Design review of the part built by this model. Coordinates are the model's own, in mm. A direction names the side the tool comes from. Round coordinates to 2 decimals unless told otherwise and drop trailing zeros. Write each loop counter-clockwise with the first axis right and the second up, starting at its lowest first coordinate (ties: lowest second). Pieces come first, ordered by that corner, then holes. Notation, with made-up numbers: M 46,33 L 101,33 A21 ccw 101,51 Z; hole C 78,4 d1. An arc over 180 degrees is marked long. One line per question, with ' | ' between items. Start each with the question number.
Item 1: Add section A-A, the plane y = 0. State the section outline as (x, z) points.
Item 2: For L1, parallel to Y at x = 0, z = 108.65; L2, parallel to Y at x = 0, z = 50; L3, parallel to Y at x = 0, z = 1.35, list the stretches that pass through material, from the lowest coordinate up.
Item 3: Insertion check: pin 1 Ø3 at (x, z) = (11, 83) entering from +Y; pin 2 Ø10 at (x, z) = (8.5, 54) entering from -Y; pin 3 Ø1 at (y, z) = (6.5, 40.5) entering from +X. Each pin has a flat end and moves straight along its axis. Give the tip position at first contact, or say it passes through.
Item 4: Add section B-B, the plane x = 0. State the section outline as (y, z) points, and give its area (3 significant figures).
Item 5: Add section D-D, the plane y = -10.25. State the section outline as (x, z) points, and give its area (3 significant figures).
Item 6: Machinability: for faces 1 (the face through (0, -7.559, 108)), 2 (the face through (-10.316, -7.91, 56.765)), 3 (the face through (3, 3.4, 110)), which of the approach directions +Z, -Z, +X, -X, +Y, -Y give a long, thin tool a straight path to every point of the face, cutting with its end or side? Answer none if there is none.
Item 7: Add section C-C, the plane z = 11.5. State the section outline as (x, y) points, and give its area (3 significant figures).
Item 8: Draft analysis for pull direction Y (two halves, no side actions). For faces 4 (the face through (2.285, 3.584, 107.535)), 5 (the face through (6.691, -12.864, 54.23)), 6 (the face through (6, 0, 5)), 7 (the face through (3, 3.4, 0)), state which applies: released by +Y, released by -Y, zero draft, split by the parting line, or undercut.
```python
from build123d import *

# Parameters (mm, degrees)
F0_R     = 14.5
F1_DEPTH = 5
F2_R     = 14.5
F2_R_2   = 13
F3_DEPTH = 105
F4_R     = 4.25
F5_DEPTH = 5
F6_R     = 4.25
F7_DEPTH = 5


with BuildPart() as f1:
    # F0 (on Top) → F1 (new body)
    with BuildSketch(Plane.XY):
        Circle(F0_R)
    extrude(amount=F1_DEPTH)

    # F2 (on face) → F3 (join)
    with BuildSketch(Plane.XY.offset(5)):
        Circle(F2_R)
        Circle(F2_R_2, mode=Mode.SUBTRACT)
    extrude(amount=F3_DEPTH)

    # F4 (on face) → F5 (cut, through all)
    with BuildSketch(Plane(origin=(0, 0, 0), x_dir=(1, 0, 0), z_dir=(0, 0, -1))):
        Circle(F4_R)
    extrude(amount=-F5_DEPTH, mode=Mode.SUBTRACT)

    # F6 (on face) → F7 (join)
    with BuildSketch(Plane.XY.offset(110)):
        with BuildLine():
            ThreePointArc((13, 0), (-3.9688128034, 12.3793588255), (-10.5766961433, -7.5586704315))
            Line((-10.5766961433, -7.5586704315), (10.5766961433, -7.5586704315))
            ThreePointArc((10.5766961433, -7.5586704315), (12.3793588255, -3.9688128034), (13, 0))
        make_face()
        Circle(F6_R, mode=Mode.SUBTRACT)
    extrude(amount=-F7_DEPTH)


solid = f1.part
```
Computed values:
1) outline: M -14.5,0 L -4.25,0 L -4.25,5 L -13,5 L -13,105 L -4.25,105 L -4.25,110 L -14.5,110 Z; M 4.25,0 L 14.5,0 L 14.5,110 L 4.25,110 L 4.25,105 L 13,105 L 13,5 L 4.25,5 Z
2) L1: y = -14.5 to -13, -7.56 to -4.25, 4.25 to 14.5 | L2: y = -14.5 to -13, 13 to 14.5 | L3: y = -14.5 to -4.25, 4.25 to 14.5
3) pin 1: stops at y = 10.95 | pin 2: stops at y = -14.07 | pin 3: stops at x = 13.2
4) outline: M -14.5,0 L -4.25,0 L -4.25,5 L -13,5 L -13,110 L -14.5,110 Z; M -7.56,105 L -4.25,105 L -4.25,110 L -7.56,110 Z; M 4.25,0 L 14.5,0 L 14.5,110 L 4.25,110 L 4.25,105 L 13,105 L 13,5 L 4.25,5 Z | area: 478 mm^2
5) outline: M -10.26,0 L 10.26,0 L 10.26,110 L 8,110 L 8,5 L -8,5 L -8,110 L -10.26,110 Z | area: 577 mm^2
6) face 1: +Z | face 2: none | face 3: +Z, +X, -X, +Y, -Y
7) outline: C 0,0 d29; hole C 0,0 d26 | area: 130 mm^2
8) face 4: undercut | face 5: split by the parting line | face 6: undercut | face 7: zero draft
